Verification items for this drawing (mm, ordinates from the low corner). A direction names the side the tool comes from. Coordinates: 2 decimals unless noted, no trailing zeros. Order: outer loops, then holes, each group sorted by start corner. A loop starts at its lowest first (then second) coordinate and runs counter-clockwise, first axis right, second up. Notation, with made-up numbers: M 42,25 L 97,25 A25 cw 97,49 Z; hole C -18.5,-22.5 d11. An arc over 180 degrees is marked long. Use CSV: the item, a comma, the result in double quotes. Start each with the question number.
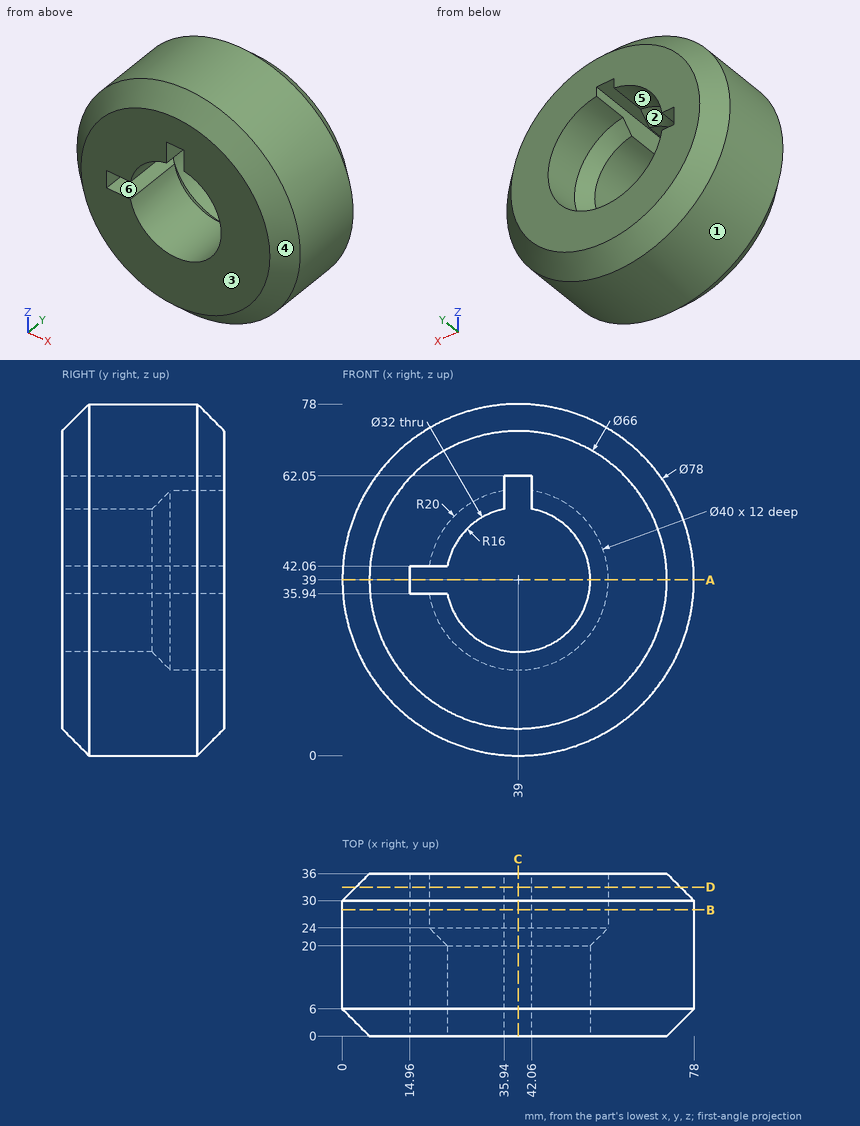
1) Material ranges on line 1 along Z through (x, y) = (39, 8); line 2 along X through (y, z) = (6.5, 39); line 3 along Z through (x, y) = (47, 28.5), recorded low to high.
2) Set-up check for the marked faces 4, 5 and 6: record each of +Z, -Z, +X, -X, +Y, -Y from which the full face is reachable in a straight line by a thin tool's end or side.
3) Section check C-C on x = 39. Record the boundary of the cut face in (y, z), then the cut area to 3 significant figures.
4) Section check A-A on z = 39. Record the boundary of the cut face in (x, y).
5) Section check B-B on y = 28. Record the boundary of the cut face in (x, z).
6) Draft check along Z on the marked faces 1, 2 and 3. Enter one of: +Z half, -Z half, draft (parallel to the pull), parting line (faces both ways), or undercut.
7) Section check D-D on y = 33. Record the boundary of the cut face in (x, z), then the cut area to 3 significant figures.
8) Gauge pin test, flat ends, axial feed: P1, Ø6, axis at y = 15, z = 62, coming from the +X side; P2, Ø1, axis at y = 8.5, z = 51.5, coming from the -X side; P3, Ø3, axis at x = 40, y = 18.5, coming from the -Z side. Record the tip position at first contact, or that the pin passes through.
Results are:
1,line 1,"z = 0 to 23, 62.05 to 78"
1,line 2,"x = 0 to 14.96, 55 to 78"
1,line 3,"z = 0.83 to 20.67, 57.33 to 77.17"
2,face 4,"-Y"
2,face 5,"+Y"
2,face 6,"+Y, -Y"
3,outline,"M 0,6 L 6,0 L 30,0 L 36,6 L 36,19 L 24,19 L 20,23 L 0,23 Z; M 0,62.05 L 36,62.05 L 36,72 L 30,78 L 6,78 L 0,72 Z"
3,area,"1,270 mm²"
4,outline,"M 0,6 L 6,0 L 14.96,0 L 14.96,36 L 6,36 L 0,30 Z; M 55,0 L 72,0 L 78,6 L 78,30 L 72,36 L 59,36 L 59,24 L 55,20 Z"
5,outline,"C 39,39 d78; hole M 14.96,35.94 L 19.24,35.94 A20 ccw long 42.06,58.76 L 42.06,62.05 L 35.94,62.05 L 35.94,58.76 A20 ccw 19.24,42.06 L 14.96,42.06 Z"
6,face 1,"parting line"
6,face 2,"undercut"
6,face 3,"draft"
7,outline,"C 39,39 d72; hole M 14.96,35.94 L 19.24,35.94 A20 ccw long 42.06,58.76 L 42.06,62.05 L 35.94,62.05 L 35.94,58.76 A20 ccw 19.24,42.06 L 14.96,42.06 Z"
7,area,"2,770 mm²"
8,P1,"stops at x = 72.48"
8,P2,"stops at x = 1.89"
8,P3,"stops at z = 0"
